Could you check a few things on this drawing? It's one solid part, dimensions in mm from its lowest x, y, z. A direction names the side the tool comes from. Give positions to 0.01 mm unless a question says otherwise; leave off trailing zeros. Loops run counter-clockwise (first coordinate to the right, second up) from the corner with the lowest first, then second, coordinate; pieces in that order, holes last. Notation, with made-up numbers: M -25.75,58 L 20.25,58 A34 ccw 20.25,88 Z; hole C -21,83 d3. An arc over 180 degrees is marked long. Answer in a Markdown table with one row per item. Add a question column.
1. Which directions (+Z, -Z, +X, -X, +Y, -Y) give clear straight access to the entire face, cutting with the end or side of a thin tool? Please do the marked faces 4, 5 and 6.
2. If we section it at D-D on z = 14: List the corners of the cut face in (x, y) for me.
3. If we section it at B-B on z = 43.5: List the corners of the cut face in (x, y) for me.
4. If we section it at A-A on x = 100: List the corners of the cut face in (y, z) for me, then the cut area to 3 significant figures.
5. Thinking about a two-plate mould opening in X: for the marked faces 1, 2 and 3, which applies, released by +X, released by -X, zero draft, split by the parting line, or undercut?
6. I need wall thicknesses on line 1 along Y through (x, z) = (20, 41.5); line 2 along Y through (x, z) = (64, 12); line 3 along X through (y, z) = (22.5, 40). Which ranges of each line are inside material? Lowest first, please. Write a range as from..to.
7. If we section it at C-C on x = 62: List the corners of the cut face in (y, z) for me.
8. I'm going to push flat-ended pins straight in: pin 1 Ø5 at (x, z) = (71.5, 37) entering from +Y; pin 2 Ø10 at (y, z) = (12, 17) entering from -X; pin 3 Ø10 at (x, z) = (48.5, 45.5) entering from -Y. Where does each tip first touch, or does it pass through?
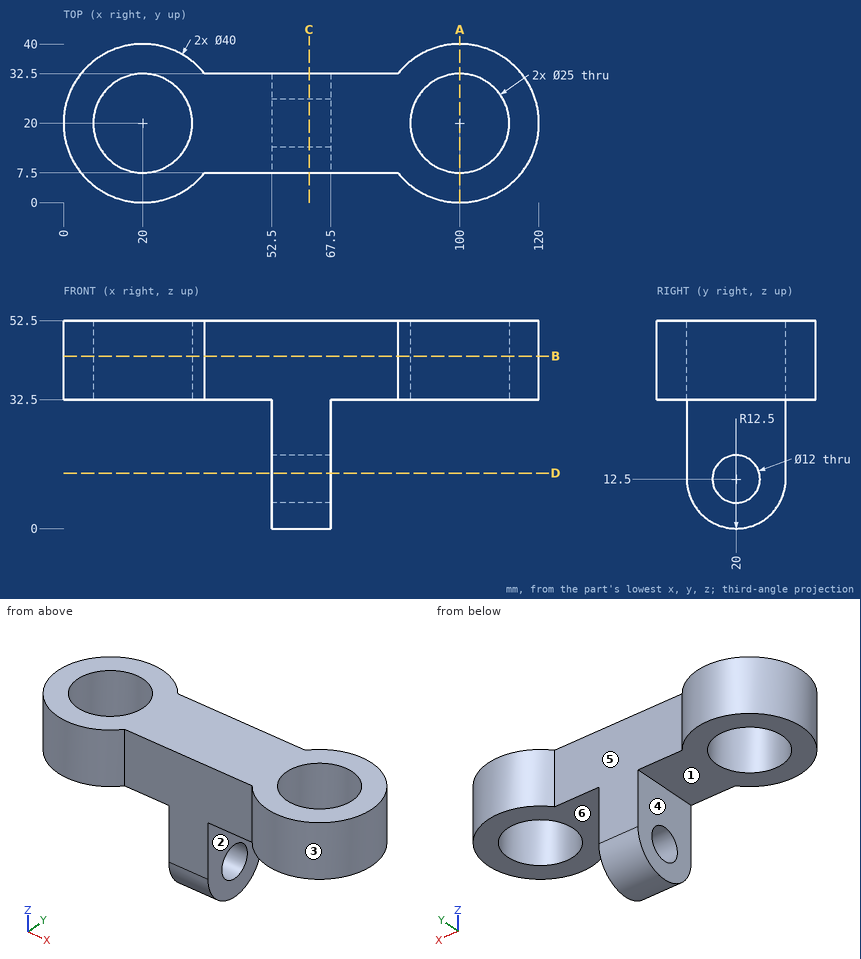
Results:
| question | item | result |
|---|---|---|
| 1 | face 4 | -Z, -X, +Y, -Y |
| 1 | face 5 | +Z, -Z, +Y |
| 1 | face 6 | -Z, +X, +Y, -Y |
| 2 | outline | M 52.5,7.5 L 67.5,7.5 L 67.5,14.19 L 52.5,14.19 Z; M 52.5,25.81 L 67.5,25.81 L 67.5,32.5 L 52.5,32.5 Z |
| 3 | outline | M 35.61,7.5 L 84.39,7.5 A20 ccw long 84.39,32.5 L 35.61,32.5 A20 ccw long Z; hole C 20,20 d25; hole C 100,20 d25 |
| 4 | outline | M 0,32.5 L 7.5,32.5 L 7.5,52.5 L 0,52.5 Z; M 32.5,32.5 L 40,32.5 L 40,52.5 L 32.5,52.5 Z |
| 4 | area | 300 mm2 |
| 5 | face 1 | zero draft |
| 5 | face 2 | released by +X |
| 5 | face 3 | undercut |
| 6 | line 1 | 0..7.5, 32.5..40 |
| 6 | line 2 | 7.51..14.02, 25.98..32.49 |
| 6 | line 3 | 0.16..7.75, 32.25..87.75, 112.25..119.84 |
| 7 | outline | M 7.5,12.5 A12.5 ccw 32.5,12.5 L 32.5,52.5 L 7.5,52.5 Z; hole C 20,12.5 d12 |
| 8 | pin 1 | y = 32.5 |
| 8 | pin 2 | x = 52.5 |
| 8 | pin 3 | y = 7.5 |
